Part model, mm, in its own coordinate system. A direction names the side the tool comes from. Round coordinates to 2 decimals unless told otherwise and drop trailing zeros. Loops run counter-clockwise (first coordinate to the right, second up) from the corner with the lowest first, then second, coordinate; pieces in that order, holes last.
1) Band-saw the part on A-A, the plane x = 16. Write the cut outline in (y, z), then the cut area to 3 significant figures.
2) Mould opens along Z. For faces 4 (the flat face through (16, -25, 23)), 5 (the flat face through (16, -31, 0)), 6 (the flat face through (28.91, -31.19, 21.48)), 7 (the flat face through (16, -20, 10)) say: +Z half, -Z half, draft (parallel to the pull), parting line (faces both ways), or undercut.
3) 3-axis set-ups, long thin cutter, end or side, ignore diameter. For faces 1 (the flat face through (16, -31, 20)), 2 (the flat face through (16, -13, -3)), 3 (the flat face through (16, 0, 17)): which of +Z, -Z, +X, -X, +Y, -Y reach the whole face in a straight line?
4) Drop a flat-ended pin along its axis: P1, Ø6, axis at x = 13, z = 10, coming from the -Y side. Give the stop position or say it passes through.
5) Band-saw the part on B-B, the plane y = -40. Write the cut outline in (x, z).
6) Band-saw the part on D-D, the plane x = 9.5. Write the cut outline in (y, z).
7) Probe line 1 (Z direction, x = 17, y = -33.5); line 2 (Y direction, x = 16, z = -1.8); line 3 (Y direction, x = 16, z = 20.9). List the from-to ranges inside material, lowest first.
8) Band-saw the part on C-C, the plane y = -27. Write the cut outline in (x, z).
Autodesk Fusion 360 part; units mm, degrees
sketch "Sketch1" plane through (0, 0, 0) normal (0, 0, 1) x (1, 0, 0)
  line L0 (0, 0) -> (32, 0)
  line L1 (0, 0) -> (0, -20)
  line L2 (0, -20) -> (32, -20)
  line L3 (32, -20) -> (32, 0)
  line L4 (16, -20) -> (16, -40) construction
  circle A0 centre (16, -40) radius 10.1
  line L5 (0, -20) -> (6.2643, -42.6881)
  line L6 (32, -20) -> (25.7357, -42.6881)
  circle A1 centre (16, -40) radius 5.1
  circle A2 centre (16, -40) radius 14 construction
  line L7 (0, -10) -> (32, -10)
  line L8 (0, 0) -> (0, 10)
  line L9 (0, 10) -> (32, 10)
  line L10 (32, 10) -> (32, 0)
  dimension "d1" = 32
  dimension "d2" = 20
  dimension "d5" = 20
  dimension "d6" = 20.2
  dimension "d7" = 10.2
  dimension "d8" = 28
  dimension "d14" = 10
extrude "Extrude1" add sketch "Sketch1" along normal blind 20 from surface at -3 contours L0 L8 L9 L10 | L0 L1 L3 L7 makes body 1
extrude "Extrude2" add sketch "Sketch1" against normal blind 3 contours L2 A0 L5 L6 | A0 bodies 1 makes body 2
extrude "Extrude3" add sketch "Sketch1" along normal blind 3 from surface at 20 contours L2 A0 L5 L6 | A0 bodies 2 makes body 3
extrude "Extrude4" add sketch "Sketch1" along normal blind 26 from surface at -3 contours L1 L2 L3 L7 bodies 1 2 3
sketch "Sketch2" plane through (0, 0, 17) normal (0, 0, 1) x (-1, 0, 0)
  line L0 (0, -10) -> (0, 10)
  line L1 (0, 10) -> (-32, 10)
  line L2 (-32, 10) -> (-32, -10)
  line L3 (-32, -10) -> (0, -10)
  line L4 (0, -10) -> (-16, -10) construction
  line L5 (-8, -10) -> (-8, 0) construction
  line L6 (-16, -10) -> (-24, -10) construction
  line L7 (-24, -10) -> (-24, 0) construction
  circle A0 centre (-24, 0) radius 1.6
  circle A1 centre (-8, 0) radius 1.6
  dimension "d19" = 8
  dimension "d20" = 10
  dimension "d21" = 3.2
  dimension "d22" = 3.2
extrude "Extrude5" cut sketch "Sketch2" along normal through all contours A0 | A1 bodies 1
equation "d9 = -( 20 / 2 ) * 2 mm + ( ( 14 + 1.5 * 2 ) / 2 ) * 2 mm"
equation "d12 = ( ( 20 / 2 ) * 2 mm - ( ( 14 + 1.5 * 2 ) / 2 ) * 2 mm )"
Reported:
1. outline: (-50.1, -3) - (-45.1, -3) - (-45.1, 0) - (-50.1, 0) - close; (-50.1, 20) - (-45.1, 20) - (-45.1, 23) - (-50.1, 23) - close; (-34.9, -3) - (10, -3) - (10, 17) - (-10, 17) - (-10, 23) - (-34.9, 23) - (-34.9, 20) - (-20, 20) - (-20, 0) - (-34.9, 0) - close
1. area: 779 mm2
2. face 4: +Z half
2. face 5: undercut
2. face 6: draft
2. face 7: undercut
3. face 1: +X, -X, -Y
3. face 2: -Z, +X, -X, +Y, -Y
3. face 3: +Z, +X, -X, +Y
4. P1: stops at y = -20
5. outline: (5.52, -3) - (10.9, -3) - (10.9, 0) - (5.52, 0) - close; (5.52, 20) - (10.9, 20) - (10.9, 23) - (5.52, 23) - close; (21.1, -3) - (26.48, -3) - (26.48, 0) - (21.1, 0) - close; (21.1, 20) - (26.48, 20) - (26.48, 23) - (21.1, 23) - close
6. outline: (-47.73, -3) - (10, -3) - (10, 17) - (-10, 17) - (-10, 23) - (-47.73, 23) - (-47.73, 20) - (-20, 20) - (-20, 0) - (-47.73, 0) - close
7. line 1: z = -3 to 0, 20 to 23
7. line 2: y = -50.1 to -45.1, -34.9 to 10
7. line 3: y = -50.1 to -45.1, -34.9 to -10
8. outline: (1.93, -3) - (30.07, -3) - (30.07, 0) - (1.93, 0) - close; (1.93, 20) - (30.07, 20) - (30.07, 23) - (1.93, 23) - close
